Build history of the part. All positions in model axes, mm. Round coordinates to 2 decimals unless told otherwise and drop trailing zeros. Write each loop counter-clockwise with the first axis right and the second up, starting at its lowest first coordinate (ties: lowest second). Pieces come first, ordered by that corner, then holes. Notation, with made-up numbers: M 71,54 L 90,54 A10 ccw 90,63 Z; hole C 58.5,-27 d10. An arc over 180 degrees is marked long. Write item = value, one per line.
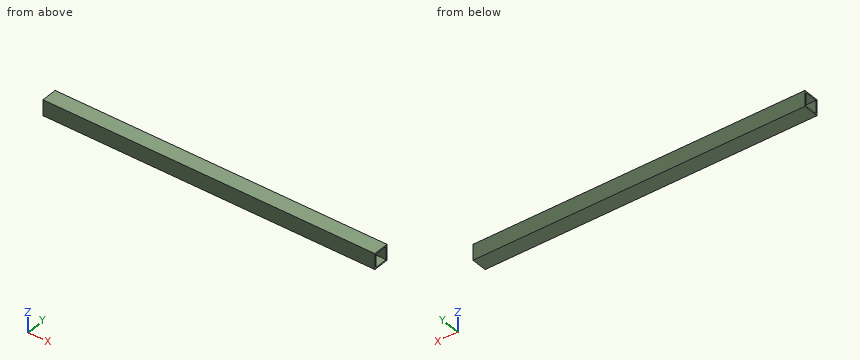
from build123d import *

# Parameters (mm, degrees)
F0_W     = 20
F0_H     = 20
F0_W_2   = 16.8
F0_H_2   = 16.8
F1_DEPTH = 212


with BuildPart() as f1:
    # F0 (on Right) → F1 (new body, symmetric)
    with BuildSketch(Plane.YZ):
        with Locations((10, -10)):
            Rectangle(F0_W, F0_H)
        with Locations((10, -10)):
            Rectangle(F0_W_2, F0_H_2, mode=Mode.SUBTRACT)
    extrude(amount=F1_DEPTH, both=True)


solid = f1.part
1. Band-saw the part on C-C (x = 136.5). List the corners of the cut face in (y, z), plus the area to 3 significant figures.
Responses:
outline = M 0,-20 L 20,-20 L 20,0 L 0,0 Z; hole M 1.6,-18.4 L 18.4,-18.4 L 18.4,-1.6 L 1.6,-1.6 Z
area = 118 mm²
2. Probe probe 1 along Z at (x, y) = (-60.5, 15.5); probe 2 along Y at (x, z) = (192.5, -6). List the from-to ranges inside material, lowest first.
Responses:
probe_1 = -20 to -18.4, -1.6 to 0
probe_2 = 0 to 1.6, 18.4 to 20
3. Band-saw the part on A-A (y = 5.5). List the corners of the cut face in (x, z), plus the area to 3 significant figures.
Responses:
outline = M -212,-20 L 212,-20 L 212,-18.4 L -212,-18.4 Z; M -212,-1.6 L 212,-1.6 L 212,0 L -212,0 Z
area = 1,360 mm²
4. Band-saw the part on B-B (z = -6). List the corners of the cut face in (x, y).
Responses:
outline = M -212,0 L 212,0 L 212,1.6 L -212,1.6 Z; M -212,18.4 L 212,18.4 L 212,20 L -212,20 Z
